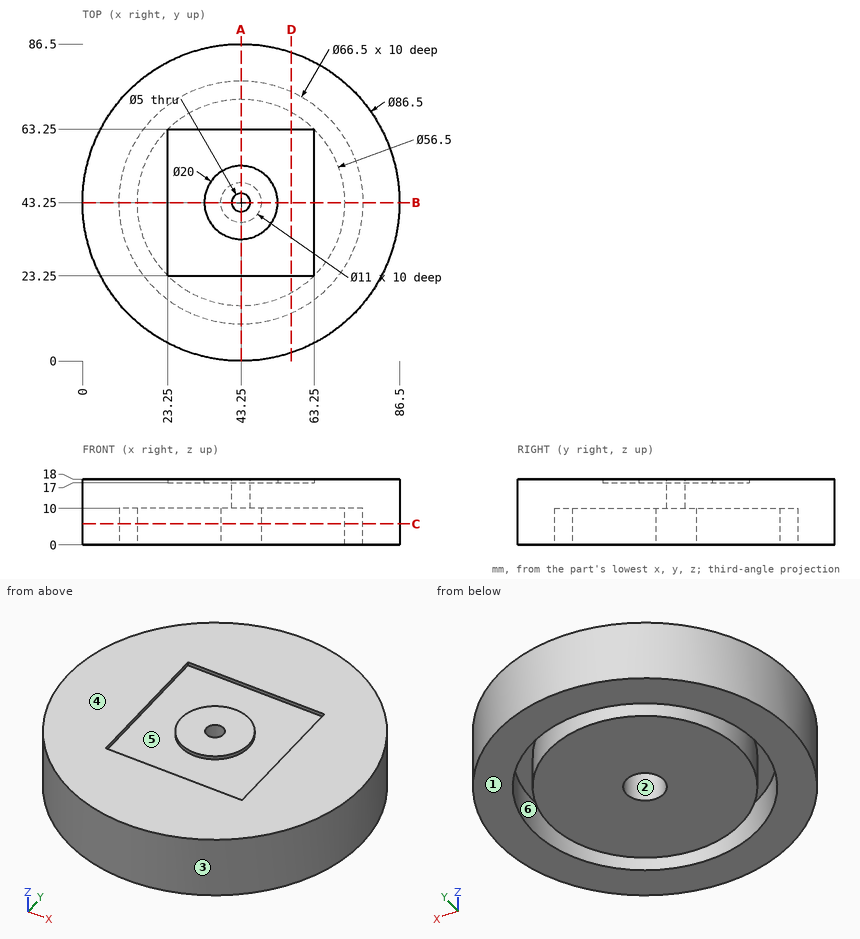
Print and shaded views of the part. All mm, measured from the part's lowest x, y and z. A direction names the side the tool comes from. Round coordinates to 2 decimals unless told otherwise and drop trailing zeros. Order: outer loops, then holes, each group sorted by start corner. A loop starts at its lowest first (then second) coordinate and runs counter-clockwise, first axis right, second up.
Q1. Slice it at D-D (x = 57). Write the cut outline in (y, z).
Q2. Drop flat-ended pins along their axis: pin 1 (4 mm diameter, centred on x = 43.25, y = 43.25, fed in from +Z); pin 2 (4 mm diameter, centred on y = 35.5, z = 11.5, fed in from +X); pin 3 (1 mm diameter, centred on x = 28.5, z = 4.5, fed in from +Y); pin 4 (6 mm diameter, centred on x = 9, z = 14.5, fed in from +Y). Give the stop position or say it passes through.
Q3. Two-plate mould, pull along Y, no slides. Class the marked faces 1, 2 and 3: pulls with the +Y half, pulls with the -Y half, needs draft (parallel to the pull), parting line crosses it, or undercut.
Q4. Which spindle directions (+Z, -Z, +X, -X, +Y, -Y) get a long thin tool onto all of the face, cutting with end or side? Do the marked faces 4, 5 and 6. Say none if no direction does.
Q5. Slice it at C-C (z = 5.75). Write the cut outline in (x, y).
Q6. Slice it at A-A (x = 43.25). Write the cut outline in (y, z), and give its area (3 significant figures).
Q7. Wall check: L1, parallel to X at y = 43.25, z = 5.5; L2, parallel to Y at x = 23, z = 5. Give the ranges that are in metal, low to high.
Results below:
1. outline: (2.24, 0) - (12.98, 0) - (12.98, 10) - (18.57, 10) - (18.57, 0) - (67.93, 0) - (67.93, 10) - (73.52, 10) - (73.52, 0) - (84.26, 0) - (84.26, 18) - (63.25, 18) - (63.25, 17) - (23.25, 17) - (23.25, 18) - (2.24, 18) - close
2. pin 1: passes through
2. pin 2: stops at x = 86.12
2. pin 3: stops at y = 84.09
2. pin 4: stops at y = 73.15
3. face 1: needs draft
3. face 2: undercut
3. face 3: parting line crosses it
4. face 4: +Z, +X, -X, +Y, -Y
4. face 5: +Z
4. face 6: -Z
5. outline: circle Ø86.5 at (43.25, 43.25); circle Ø56.5 at (43.25, 43.25); hole circle Ø66.5 at (43.25, 43.25); hole circle Ø11 at (43.25, 43.25)
6. outline: (0, 0) - (10, 0) - (10, 10) - (15, 10) - (15, 0) - (37.75, 0) - (37.75, 10) - (40.75, 10) - (40.75, 18) - (33.25, 18) - (33.25, 17) - (23.25, 17) - (23.25, 18) - (0, 18) - close; (45.75, 10) - (48.75, 10) - (48.75, 0) - (71.5, 0) - (71.5, 10) - (76.5, 10) - (76.5, 0) - (86.5, 0) - (86.5, 18) - (63.25, 18) - (63.25, 17) - (53.25, 17) - (53.25, 18) - (45.75, 18) - close
6. area: 1,290 mm2
7. L1: x = 0 to 10, 15 to 37.75, 48.75 to 71.5, 76.5 to 86.5
7. L2: y = 5.03 to 16.88, 23.55 to 62.95, 69.62 to 81.47
